Could you check a few things on this drawing? It's one solid part, dimensions in mm from its lowest x, y, z. Round coordinates to 2 decimals unless told otherwise and drop trailing zeros. Write each loop counter-clockwise with the first axis right and the second up, starting at its lowest first coordinate (ties: lowest second). Pieces come first, ordered by that corner, then holes. Notation, with made-up numbers: (85, 84) -> (126, 84) arc R36 ccw to (126, 123) -> close; hole circle Ø11 at (-11.5, 15). An arc over 180 degrees is marked (long way). Answer in a Markdown table with one row per item. Add a question column.
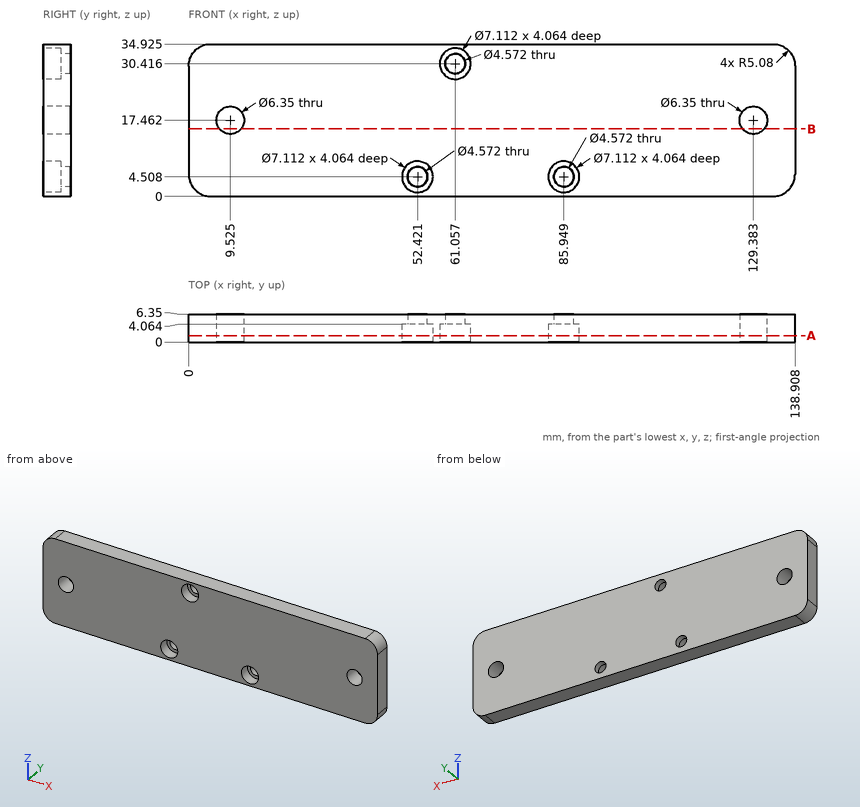
Item 1: I need wall thicknesses on line 1 along X through (y, z) = (3.75, 3.5) (1 decimal); line 2 along X through (y, z) = (4.5, 16) (1 decimal); line 3 along Z through (x, y) = (9.5, 4.5) (1 decimal). Which ranges of each line are inside material? Lowest first, please. Write a range as from..to.
Item 2: For P1, Ø4, axis at x = 129.38, z = 17.46, coming from the -Y side; P2, Ø3.5, axis at x = 54, z = 4, coming from the -Y side; P3, Ø3, axis at x = 39.5, y = 5.5, coming from the -Z side, each with a flat end and sliding along its axis, tell me the tip position at first contact or that it passes through.
Item 3: If we section it at B-B on z = 15.5: Please give me the cut outline in (x, y).
Item 4: If we section it at A-A on y = 1.5: Give the number of separate pieces and of enclosed holes in the cut face, then the cut area to 3 significant figures.
Results list:
| question | item | result |
|---|---|---|
| 1 | line 1 | 0.3..49, 55.8..82.5, 89.4..138.7 |
| 1 | line 2 | 0..6.7, 12.3..126.6, 132.2..138.9 |
| 1 | line 3 | 0..14.3, 20.6..34.9 |
| 2 | P1 | through |
| 2 | P2 | y = 4.06 |
| 2 | P3 | z = 0 |
| 3 | outline | (0, 0) -> (7.03, 0) -> (7.03, 6.35) -> (0, 6.35) -> close; (12.02, 0) -> (126.89, 0) -> (126.89, 6.35) -> (12.02, 6.35) -> close; (131.88, 0) -> (138.91, 0) -> (138.91, 6.35) -> (131.88, 6.35) -> close |
| 4 | separate pieces | 1 |
| 4 | enclosed holes | 5 |
| 4 | area | 4,650 mm² |
